Could you check a few things on this model? Use its own coordinates, in mm. A direction names the side the tool comes from. Give positions to 0.01 mm unless a question says otherwise; leave off trailing zeros. Order: outer loops, then holes, each group sorted by start corner. A loop starts at its lowest first (then second) coordinate and runs counter-clockwise, first axis right, second up. Notation, with made-up numbers: (15, -25) - (55, -25) arc R21 ccw to (55, -4) - close; hole circle Ø3 at (16, 80.25). An arc over 180 degrees is marked (long way). Put each result on its own line as item: value.
from build123d import *
from build123d import SkipClean  # not in build123d's __all__

# Parameters (mm, degrees)
F0_W     = 58.7
F0_H     = 31.916891567
F0_W_2   = 50.8
F0_H_2   = 17.5
F0_W_3   = 1.3
F0_H_3   = 0.083108433
F1_DEPTH = 25
F2_D     = 5.4102
F3_DEPTH = 25


with BuildPart() as f1:
    # F0 (on Top) → F1 (new body)
    with BuildSketch(Plane.XY):
        with BuildLine():
            ThreePointArc((0, 3.5), (2.4748737342, 2.4748737342), (3.5, 0))
            Line((3.5, 0), (79.5, 0))
            Line((79.5, 0), (79.5, 36.256108433))
            Line((79.5, 36.256108433), (58.7, 36.256108433))
            Line((58.7, 36.256108433), (58.7, 36.173))
            Line((58.7, 36.173), (0, 36.173))
            Line((0, 36.173), (0, 3.5))
        make_face()
        with BuildLine():
            Line((58.7, 36.256108433), (79.5, 36.256108433))
            Line((79.5, 36.256108433), (79.5, 42.475))
            ThreePointArc((79.5, 42.475), (76, 45.975), (79.5, 49.475))
            Line((79.5, 49.475), (79.5, 87.056108433))
            Line((79.5, 87.056108433), (0, 87.056108433))
            Line((0, 87.056108433), (0, 79.6536390185))
            ThreePointArc((0, 79.6536390185), (1.4142135624, 79.0678525809), (2, 77.6536390185))
            ThreePointArc((2, 77.6536390185), (1.4142135624, 76.2394254562), (0, 75.6536390185))
            Line((0, 75.6536390185), (0, 68.173))
            Line((0, 68.173), (58.7, 68.173))
            Line((58.7, 68.173), (58.7, 36.256108433))
        make_face()
        with Locations((29.35, 52.2145542165)):
            Rectangle(F0_W, F0_H)
        with Locations((28.7, 52.173)):
            Rectangle(F0_W_2, F0_H_2, mode=Mode.SUBTRACT)
        with BuildLine():
            Line((79.5, 0), (3.5, 0))
            ThreePointArc((3.5, 0), (-2.4748737342, -2.4748737342), (0, 3.5))
            Line((0, 3.5), (0, 36.173))
            Line((0, 36.173), (-1.3, 36.173))
            Line((-1.3, 36.173), (-1.3, 36.256108433))
            Line((-1.3, 36.256108433), (-4.48, 36.256108433))
            Line((-4.48, 36.256108433), (-4.48, -8.1671467051))
            Line((-4.48, -8.1671467051), (84.52, -8.1671467051))
            Line((84.52, -8.1671467051), (84.52, 36.256108433))
            Line((84.52, 36.256108433), (79.5, 36.256108433))
            Line((79.5, 36.256108433), (79.5, 0))
        make_face()
        with Locations((28.7, 52.173)):
            Rectangle(F0_W_2, F0_H_2)
        with BuildLine():
            Line((79.5, 87.056108433), (84.52, 87.056108433))
            Line((84.52, 87.056108433), (84.52, 100.6101816893))
            Line((84.52, 100.6101816893), (28.7, 100.6101816893))
            Line((28.7, 100.6101816893), (-4.48, 100.6101816893))
            Line((-4.48, 100.6101816893), (-4.48, 87.056108433))
            Line((-4.48, 87.056108433), (0, 87.056108433))
            Line((0, 87.056108433), (0, 88.45))
            ThreePointArc((0, 88.45), (-2.4748737342, 94.4248737342), (3.5, 91.95))
            Line((3.5, 91.95), (79.5, 91.95))
            Line((79.5, 91.95), (79.5, 87.056108433))
        make_face()
        with BuildLine():
            Line((0, 87.056108433), (79.5, 87.056108433))
            Line((79.5, 87.056108433), (79.5, 91.95))
            Line((79.5, 91.95), (3.5, 91.95))
            ThreePointArc((3.5, 91.95), (2.4748737342, 89.4751262658), (0, 88.45))
            Line((0, 88.45), (0, 87.056108433))
        make_face()
        with BuildLine():
            Line((79.5, 42.475), (79.5, 36.256108433))
            Line((79.5, 36.256108433), (84.52, 36.256108433))
            Line((84.52, 36.256108433), (84.52, 87.056108433))
            Line((84.52, 87.056108433), (79.5, 87.056108433))
            Line((79.5, 87.056108433), (79.5, 49.475))
            ThreePointArc((79.5, 49.475), (81.9748737342, 48.4498737342), (83, 45.975))
            ThreePointArc((83, 45.975), (81.9748737342, 43.5001262658), (79.5, 42.475))
        make_face()
        with BuildLine():
            Line((-1.3, 68.173), (0, 68.173))
            Line((0, 68.173), (0, 75.6536390185))
            ThreePointArc((0, 75.6536390185), (-2, 77.6536390185), (0, 79.6536390185))
            Line((0, 79.6536390185), (0, 87.056108433))
            Line((0, 87.056108433), (-4.48, 87.056108433))
            Line((-4.48, 87.056108433), (-4.48, 36.256108433))
            Line((-4.48, 36.256108433), (-1.3, 36.256108433))
            Line((-1.3, 36.256108433), (-1.3, 68.173))
        make_face()
        with Locations((-0.65, 52.2145542165)):
            Rectangle(F0_W_3, F0_H)
        with Locations((29.35, 36.2145542165)):
            Rectangle(F0_W, F0_H_3)
        with Locations((-0.65, 36.2145542165)):
            Rectangle(F0_W_3, F0_H_3)
    extrude(amount=-F1_DEPTH)

    # F2 (through all)
    with Locations(Plane.XY):
        with Locations((3.3, 60.923), (3.3, 43.423), (54.1, 43.423), (54.1, 60.923)):
            Hole(F2_D / 2)

    # F0 (on Top) → F3 (join)
    with BuildSketch(Plane.XY):
        with BuildLine():
            Line((-1.3, 68.173), (0, 68.173))
            Line((0, 68.173), (0, 75.6536390185))
            ThreePointArc((0, 75.6536390185), (-2, 77.6536390185), (0, 79.6536390185))
            Line((0, 79.6536390185), (0, 87.056108433))
            Line((0, 87.056108433), (-4.48, 87.056108433))
            Line((-4.48, 87.056108433), (-4.48, 36.256108433))
            Line((-4.48, 36.256108433), (-1.3, 36.256108433))
            Line((-1.3, 36.256108433), (-1.3, 68.173))
        make_face()
        with BuildLine():
            Line((58.7, 36.256108433), (79.5, 36.256108433))
            Line((79.5, 36.256108433), (79.5, 42.475))
            ThreePointArc((79.5, 42.475), (76, 45.975), (79.5, 49.475))
            Line((79.5, 49.475), (79.5, 87.056108433))
            Line((79.5, 87.056108433), (0, 87.056108433))
            Line((0, 87.056108433), (0, 79.6536390185))
            ThreePointArc((0, 79.6536390185), (1.4142135624, 79.0678525809), (2, 77.6536390185))
            ThreePointArc((2, 77.6536390185), (1.4142135624, 76.2394254562), (0, 75.6536390185))
            Line((0, 75.6536390185), (0, 68.173))
            Line((0, 68.173), (58.7, 68.173))
            Line((58.7, 68.173), (58.7, 36.256108433))
        make_face()
        with Locations((-0.65, 52.2145542165)):
            Rectangle(F0_W_3, F0_H)
    with SkipClean():  # cleaning this boolean's faces spoils the solid; the shape is the same uncleaned
        extrude(amount=F3_DEPTH)


solid = f1.part
1) We'd pull the mould along Y, two halves only. Please class faces 6 (the cylindrical face through (3.886, 58.282, -12.675)), 7 (the flat face through (29, 68.173, 12)), 8 (the flat face through (58.7, 52, 12)): pulls with the +Y half, pulls with the -Y half, needs draft (parallel to the pull), parting line crosses it, or undercut.
Filled in:
face 6: undercut
face 7: pulls with the -Y half
face 8: needs draft
2) Suppose I cut it at B-B, the plane y = 39.5. List the corners of the cut face in (x, z) for me, and give its area (3 significant figures).
Filled in:
outline: (-4.48, -25) - (84.52, -25) - (84.52, 0) - (79.5, 0) - (79.5, 25) - (58.7, 25) - (58.7, 0) - (0, 0) - (0, 25) - (-4.48, 25) - close
area: 2,860 mm^2
3) If I drill on line 1 (Y direction, x = 54.1, z = -9); line 2 (X direction, y = 51.5, z = 17); line 3 (X direction, y = 0, z = -19), over which ranges is the centre line in solid material (lowest first)? Write a range as [from, to].
Filled in:
line 1: y = [-8.17, 40.72], [46.13, 58.22], [63.63, 100.61]
line 2: x = [-4.48, 0], [58.7, 79.5]
line 3: x = [-4.48, -3.5], [3.5, 84.52]
4) I'm going to push flat-ended pins straight in: pin 1 (2 mm diameter, centred on x = 73, z = 11, fed in from +Y); pin 2 (9 mm diameter, centred on x = 0, y = 91.95, fed in from +Z); pin 3 (23 mm diameter, centred on x = 72, z = 8, fed in from -Y); pin 4 (5 mm diameter, centred on y = 40.5, z = 6.5, fed in from +X). Where does each tip first touch, or does it pass through?
Filled in:
pin 1: stops at y = 87.06
pin 2: stops at z = 0
pin 3: stops at y = -8.17
pin 4: stops at x = 79.5
5) Suppose I cut it at C-C, the plane y = 90.5. List the corners of the cut face in (x, z) for me.
Filled in:
outline: (-4.48, -25) - (-3.19, -25) - (-3.19, 0) - (-4.48, 0) - close; (3.19, -25) - (84.52, -25) - (84.52, 0) - (3.19, 0) - close
6) Suppose I cut it at A-A, the plane z = 3.5. List the corners of the cut face in (x, y) for me (3 decimals).
Filled in:
outline: (-4.48, 36.256) - (0, 36.256) - (0, 68.173) - (58.7, 68.173) - (58.7, 36.256) - (79.5, 36.256) - (79.5, 42.475) arc R3.5 cw to (79.5, 49.475) - (79.5, 87.056) - (-4.48, 87.056) - close; hole circle Ø4 at (0, 77.654)
7) Suppose I cut it at D-D, the plane x = 19.5. List the corners of the cut face in (y, z) for me.
Filled in:
outline: (-8.17, -25) - (100.61, -25) - (100.61, 0) - (87.06, 0) - (87.06, 25) - (68.17, 25) - (68.17, 0) - (-8.17, 0) - close
8) Which directions (+Z, -Z, +X, -X, +Y, -Y) give clear straight access to the entire face, cutting with the end or side of a thin tool? Please do faces 1 (the flat face through (69, 36.256, 12)), 2 (the flat face through (38, 87.056, 12)), 3 (the cylindrical face through (54.5, 46.1, -12.7)), 4 (the flat face through (79.5, 68, 12)), 5 (the flat face through (0, 52, 12)).
Filled in:
face 1: +Z, +X, -X, -Y
face 2: +Z, +X, -X, +Y
face 3: +Z, -Z
face 4: +Z, +X, +Y, -Y
face 5: +Z, -Y
